Verification items for the finished model (mm, model axes). A direction names the side the tool comes from. Round coordinates to 2 decimals unless told otherwise and drop trailing zeros. Order: outer loops, then holes, each group sorted by start corner. A loop starts at its lowest first (then second) coordinate and runs counter-clockwise, first axis right, second up. Notation, with made-up numbers: (52.5, -15.75) -> (80.5, -15.75) arc R16 ccw to (80.5, 6.25) -> close; hole circle Ø4 at (46.25, 63). An arc over 180 degrees is marked (long way). Answer in a Markdown table with one row per item. Add a question column.
```python
from build123d import *

# Parameters (mm, degrees)
SKETCH1_W               = 8
SKETCH1_H               = 8
BOSS_EXTRUDE1_DEPTH     = 3
CUT_EXTRUDE1_DEPTH      = 12.704699911
CUT_EXTRUDE1_DEPTH_BACK = 12.704699911
CUT_EXTRUDE2_DEPTH      = 11
SKETCH4_R               = 1.8
CUT_EXTRUDE3_DEPTH      = 0.8
SKETCH5_W               = 8
SKETCH5_H               = 1
BOSS_EXTRUDE2_DEPTH     = 2
FILLET1_R               = 4
CUT_EXTRUDE4_DEPTH      = 0.4


with BuildPart() as part:
    # Sketch1 → Boss-Extrude1 (new body)
    with BuildSketch(Plane(origin=(0, 0, 0), x_dir=(1, 0, 0), z_dir=(0, 1, 0))):
        with Locations((4, 4)):
            Rectangle(SKETCH1_W, SKETCH1_H)
    extrude(amount=BOSS_EXTRUDE1_DEPTH)

    # Sketch2 → Cut-Extrude1 (cut, two sides: drawn at the far end of the back side and taken through both)
    with BuildSketch(Plane.XY.offset(-CUT_EXTRUDE1_DEPTH_BACK)):
        Polygon((0, 0), (0.6, 3), (0, 3), align=None)
        Polygon((8, 0), (7.4, 3), (8, 3), align=None)
    extrude(amount=CUT_EXTRUDE1_DEPTH + CUT_EXTRUDE1_DEPTH_BACK, mode=Mode.SUBTRACT)

    # Sketch3 → Cut-Extrude2 (cut)
    with BuildSketch(Plane(origin=(0, 0, 0), x_dir=(0, 0, -1), z_dir=(1, 0, 0))):
        Polygon((0, 0), (0.6, 3), (0, 3), align=None)
        Polygon((8, 3), (7.4, 3), (8, 0), align=None)
    extrude(amount=CUT_EXTRUDE2_DEPTH, mode=Mode.SUBTRACT)

    # Sketch4 → Cut-Extrude3 (cut)
    with BuildSketch(Plane.XZ):
        with Locations(Location((4, -3.75, 0), (0, 0, 270))):
            Circle(SKETCH4_R)
    extrude(amount=-CUT_EXTRUDE3_DEPTH, mode=Mode.SUBTRACT)

    # Sketch5 → Boss-Extrude2 (add)
    with BuildSketch(Plane.XZ):
        with Locations((4, -7.5)):
            Rectangle(SKETCH5_W, SKETCH5_H)
    extrude(amount=BOSS_EXTRUDE2_DEPTH)

    # Fillet1
    # the kernel refuses this fillet: 4 mm, written as the material it takes off along each edge
    with BuildSketch(Plane(origin=(8, -2, -16.660254038), x_dir=(0, 1, 0), z_dir=(0, 0, 1)), Plane(origin=(0, -2, 1.660254038), x_dir=(0, 1, 0), z_dir=(0, 0, -1))) as fillet1_piece_1:
        with BuildLine():
            CenterArc((4, 3.464101615), FILLET1_R, 180, 60)
            Line((0, 3.464101615), (-0.08, 3.464101615))
            Line((-0.08, 3.464101615), (-0.08, 0))
            Line((-0.08, 0), (0, -0.08))
            ThreePointArc((0, -0.08), (1, -0.08), (1.96, -0.069282032))
            Line((1.96, -0.069282032), (2, 0))
        make_face()
    extrude(amount=18.320508076, mode=Mode.SUBTRACT)

    # Sketch6 → Cut-Extrude4 (cut)
    with BuildSketch(Plane(origin=(0, 3, 0), x_dir=(1, 0, 0), z_dir=(0, 1, 0))):
        with BuildLine():
            Line((2.413140262, 5.995145478), (3.182371031, 5.995145478))
            Line((3.182371031, 5.995145478), (3.182371031, 3.824472401))
            add(Edge.make_bspline(
                [(3.182371031, 3.824472401), (3.182664695, 3.783339968), (3.183225327, 3.704814249), (3.183611242, 3.59262518), (3.18574694, 3.491896749), (3.190378411, 3.402466647), (3.193557117, 3.32438048), (3.199459629, 3.257623918), (3.205347836, 3.202222959), (3.211072588, 3.16927001), (3.213621031, 3.154600607)],
                knots=[0, 0, 0, 0, 1.470600056, 2.807515117, 4.011048972, 5.072079398, 6.00911328, 6.804506435, 7.467811572, 8, 8, 8, 8], degree=3))
            add(Edge.make_bspline(
                [(3.213621031, 3.154600607), (3.224127628, 3.115054038), (3.244816443, 3.03718185), (3.301842427, 2.930732637), (3.377172946, 2.83690436), (3.454012852, 2.769989694), (3.523520467, 2.722632459), (3.582561491, 2.693810163), (3.645203631, 2.667536787), (3.712771176, 2.647377448), (3.784538951, 2.629737301), (3.861373833, 2.619537644), (3.942627383, 2.611709661), (3.998321517, 2.610930314), (4.026922313, 2.610530094)],
                knots=[0, 0, 0, 0, 1.376921055, 2.711331395, 4.038631339, 5.418057255, 6.132954575, 6.870556231, 7.630397752, 8.422890386, 9.247036838, 10.121396817, 11.035274583, 12, 12, 12, 12], degree=3))
            add(Edge.make_bspline(
                [(4.026922313, 2.610530094), (4.055777389, 2.611053435), (4.111957634, 2.612072369), (4.193372399, 2.618140476), (4.269330983, 2.629588903), (4.339786919, 2.644600001), (4.40511233, 2.663571514), (4.464786061, 2.687591678), (4.518714075, 2.716497769), (4.582078678, 2.760066391), (4.650258908, 2.821527538), (4.715873674, 2.905091818), (4.762833649, 2.997337694), (4.784859868, 3.081565077), (4.796180605, 3.154949811), (4.803077806, 3.219164001), (4.809385646, 3.291832182), (4.815113647, 3.372755319), (4.819030865, 3.461994153), (4.821149619, 3.559774375), (4.82281709, 3.666080391), (4.823198873, 3.739802878), (4.823396672, 3.777998042)],
                knots=[0, 0, 0, 0, 1.036876239, 2.018776863, 2.930845756, 3.794842666, 4.605604932, 5.371924355, 6.101864688, 6.799283669, 8.1310906, 9.382718023, 10.597336334, 11.822035891, 12.492591141, 13.265194674, 14.141890321, 15.11351293, 16.179860579, 17.351049011, 18.627594861, 20, 20, 20, 20], degree=3))
            Line((4.823396672, 3.777998042), (4.823396672, 5.995145478))
            Line((4.823396672, 5.995145478), (5.592627441, 5.995145478))
            Line((5.592627441, 5.995145478), (5.592627441, 3.902998042))
            add(Edge.make_bspline(
                [(5.592627441, 3.902998042), (5.592528847, 3.845305157), (5.592339402, 3.734449864), (5.589381475, 3.574956755), (5.583094941, 3.428628514), (5.577830511, 3.295214312), (5.567675642, 3.175054503), (5.557043529, 3.068074376), (5.543346947, 2.974292627), (5.523815493, 2.867696041), (5.490991615, 2.748101531), (5.438090809, 2.615994056), (5.370481989, 2.495804532), (5.288434562, 2.387071806), (5.192421188, 2.289363714), (5.081004269, 2.203064381), (4.955329501, 2.127124651), (4.84016309, 2.072443299), (4.739752735, 2.035622669), (4.65797018, 2.010704116), (4.570444093, 1.989952175), (4.477277128, 1.973483664), (4.378429252, 1.959598273), (4.273864574, 1.950325107), (4.163741291, 1.944537997), (4.088628699, 1.944091898), (4.050159493, 1.943863427)],
                knots=[0, 0, 0, 0, 1.415574045, 2.719986624, 3.913607924, 5.00929969, 5.995467356, 6.871900228, 7.64671288, 8.320227872, 9.530145585, 10.682614022, 11.803571353, 12.90325401, 14.015460715, 15.154679255, 16.351678057, 17.612271512, 18.275764165, 18.974412946, 19.708786676, 20.481351116, 21.295095879, 22.157200529, 23.056203067, 24, 24, 24, 24], degree=3))
            add(Edge.make_bspline(
                [(4.050159493, 1.943863427), (4.00394899, 1.944454117), (3.914432357, 1.945598373), (3.784491522, 1.950702797), (3.663419731, 1.961238523), (3.550836598, 1.975478544), (3.446788608, 1.993784557), (3.351012543, 2.015669281), (3.264273035, 2.043328483), (3.160959321, 2.082832512), (3.045798952, 2.143260432), (2.920442018, 2.223870786), (2.810400187, 2.314853884), (2.716640343, 2.415320705), (2.638260762, 2.521740618), (2.574552012, 2.631810814), (2.523497916, 2.743696672), (2.502164616, 2.821459533), (2.491665903, 2.859728812)],
                knots=[0, 0, 0, 0, 1.128613534, 2.186292659, 3.174878439, 4.095586888, 4.95671962, 5.754129884, 6.492676435, 7.178284149, 8.453103036, 9.659838108, 10.813193309, 11.929983019, 13.007587775, 14.033493319, 15.032227051, 16, 16, 16, 16], degree=3))
            add(Edge.make_bspline(
                [(2.491665903, 2.859728812), (2.48524032, 2.889857793), (2.471705989, 2.953319061), (2.456334745, 3.054210037), (2.442311642, 3.165307899), (2.432733679, 3.286744058), (2.423654648, 3.418133217), (2.417136225, 3.559723113), (2.414455843, 3.711481594), (2.413587623, 3.816192051), (2.413140262, 3.870145478)],
                knots=[0, 0, 0, 0, 0.728071598, 1.533551606, 2.411422299, 3.374601532, 4.412367648, 5.524718474, 6.72457895, 8, 8, 8, 8], degree=3))
            Line((2.413140262, 3.870145478), (2.413140262, 5.995145478))
        make_face()
    extrude(amount=-CUT_EXTRUDE4_DEPTH, mode=Mode.SUBTRACT)


solid = part.part
```
1) Depth check by flat-ended pin: P1, Ø1, axis at x = 5.5, z = -3, coming from the -Y side; P2, Ø1, axis at y = 1, z = -4.5, coming from the +X side; P3, Ø1.8, axis at x = 4.5, z = -3.5, coming from the -Y side. Enter the tip coordinate at first touch or a pass-through.
2) Tool access check on faces 5 (the face through (4, -1, -7)), 6 (the face through (7.7, 1.5, -4.1)), 7 (the face through (4.541, 0.394, -5.467)). Record the directions out of +Z, -Z, +X, -X, +Y, -Y that give a thin tool (end or side, any length) a straight path to the whole face; none if there is none.
3) Cross-section at A-A, the plane z = -1. Record the boundary of the cut face in (x, y), and give its area (3 significant figures).
4) Draft check along X on faces 1 (the face through (3, 0, -2)), 2 (the face through (4, 0.8, -4)), 3 (the face through (1.49, -1.48, -7.49)), 4 (the face through (3, 2.6, -4)). Enter one of: +X half, -X half, draft (parallel to the pull), parting line (faces both ways), or undercut.
5) Thickness scan on L1, parallel to Y at x = 5.25, z = -2.5; L2, parallel to Y at x = 6.75, z = -5.25; L3, parallel to X at y = 0.65, z = -4. Record the ranges inside material, lowest first. Write a range as [from, to].
6) Cross-section at B-B, the plane y = 1.7. Record the boundary of the cut face in (x, z).
Results below:
| question | item | result |
|---|---|---|
| 1 | P1 | y = 0 |
| 1 | P2 | x = 7.9 |
| 1 | P3 | y = 0.8 |
| 2 | face 5 | +Z, +X, -X, -Y |
| 2 | face 6 | +Z, -Z, +X, +Y |
| 2 | face 7 | -Y |
| 3 | outline | (0, 0) -> (8, 0) -> (7.4, 3) -> (0.6, 3) -> close |
| 3 | area | 22.2 mm² |
| 4 | face 1 | draft |
| 4 | face 2 | undercut |
| 4 | face 3 | -X half |
| 4 | face 4 | undercut |
| 5 | L1 | [0.8, 2.6] |
| 5 | L2 | [0, 3] |
| 5 | L3 | [0.13, 2.22], [5.78, 7.87] |
| 6 | outline | (0.34, -7.66) -> (7.66, -7.66) -> (7.66, -0.34) -> (0.34, -0.34) -> close |
